Can you work these out from the model? Positions are in its coordinate system, mm. Face numbers are marked on the shaded views. Give positions to 0.01 mm unless a question says otherwise; leave off trailing zeros. Order: outer loops, then holes, each group sorted by start corner. A loop starts at its lowest first (then second) coordinate and runs counter-clockwise, first axis right, second up. Notation, with made-up numbers: (31.25, 31.25) - (46.25, 31.25) arc R29 ccw to (46.25, 70.25) - close; hole circle Ø4 at (79, -18). An arc over 180 degrees is marked (long way). Use one line per item in the form item = value. Start each with the question number.
1) Please list where these lines run through material, in increasing order: probe 1 along Z at (x, y) = (-10, 3.7); probe 2 along X at (y, z) = (1.4, -10).
2) We'd pull the mould along Z, two halves only. Please class the marked faces 1, 2 and 3: released by +Z, released by -Z, zero draft, split by the parting line, or undercut.
3) For pin 1 (3 mm diameter, centred on x = -7.5, z = -1, fed in from -Y), with a flat end and sliding along its axis, tell me the tip position at first contact or that it passes through.
4) Suppose I cut it at A-A, the plane y = 3.55. Write out the boundary of the cut face in (x, z).
Autodesk Fusion 360 part; units mm, degrees
sketch "Skizze1" plane through (0, 0, 0) normal (0, 1, 0) x (1, 0, 0)
  line L0 (10, 10) -> (-10, 10) construction
  line L1 (-10, 10) -> (-10, -10) construction
  line L2 (-10, -10) -> (10, -10) construction
  line L3 (10, -10) -> (10, 10) construction
  line L4 (10, 10) -> (-10, -10) construction
  line L5 (-10, 10) -> (10, -10) construction
  circle A0 centre (-10, 10) radius 0.8
  circle A1 centre (10, 10) radius 0.8
  circle A2 centre (10, -10) radius 0.8
  circle A3 centre (-10, -10) radius 0.8
  line L6 (12, 12) -> (-12, 12)
  line L7 (-12, 12) -> (-12, -12)
  line L8 (-12, -12) -> (12, -12)
  line L9 (12, -12) -> (12, 12)
  line L10 (12, 12) -> (-12, -12) construction
  line L11 (-12, 12) -> (12, -12) construction
  circle A4 centre (0, 0) radius 9
  dimension "d1" = 20
  dimension "d2" = 20
  dimension "d3" = 1.6
  dimension "d4" = 24
  dimension "d16" = 18
extrude "Extrusion1" add sketch "Skizze1" along normal blind 4
sketch "Skizze2" plane through (0, 0, 12) normal (0, 0, 1) x (1, 0, 0)
  line L0 (-12, 0) -> (12, 0)
  line L1 (12, 4) -> (-12, 4)
  line L2 (-12, 4) -> (-12, 0)
  ellipse E0 centre (0, 0) end of major axis (8, 0) minor radius 2.5
  line L3 (-8, 0) -> (8, 0)
  line L4 (0, -2.5) -> (0, 2.5)
  dimension "d8" = 16
  dimension "d9" = 5
extrude "Extrusion2" cut sketch "Skizze2" against normal blind 27 contours L0 E0 L3 L4 | L0 E0 L3 L4 picked at (-4.5024, 0.6044) picked at (4.5261, 0.5973)
sketch "Skizze3" plane through (12, 0, 0) normal (1, 0, 0) x (0, 0, -1)
  line L0 (-12, 0) -> (12, 0)
  line L1 (12, 0) -> (12, 4)
  line L2 (12, 4) -> (-12, 4)
  line L3 (-12, 4) -> (-12, 0)
  ellipse E0 centre (0, 0) end of major axis (8, 0) minor radius 2.5
  line L4 (-8, 0) -> (8, 0)
  line L5 (0, -2.5) -> (0, 2.5)
  dimension "d12" = 5
  dimension "d13" = 16
extrude "Extrusion3" cut sketch "Skizze3" against normal blind 27 contours L0 E0 L4 L5 | L0 E0 L4 L5 picked at (-4.5024, 0.6044) picked at (4.5261, 0.5973)
fillet "Abrundung1" radius 2 4 edges at (12, 2, -12) (-12, 2, 12) (-12, 2, -12) (12, 2, 12)
equation "d1 = d2"
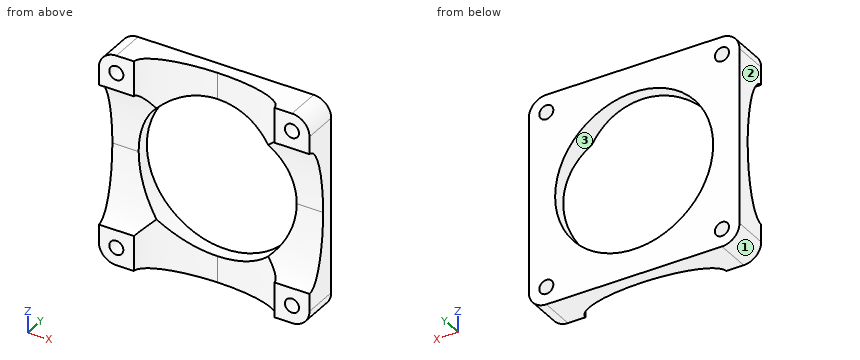
Result sheet:
q1.probe_1 = -12 to -10.8, -9.2 to 9.2, 10.8 to 12
q1.probe_2 = -12 to -10.8, -9.2 to -6.63, 6.63 to 9.2, 10.8 to 12
q2.face_1 = released by -Z
q2.face_2 = zero draft
q2.face_3 = undercut
q3.pin_1 = 2.45
q4.outline = (-12, -10) arc R2 ccw to (-10, -12) - (10, -12) arc R2 ccw to (12, -10) - (12, 10) arc R2 ccw to (10, 12) - (-10, 12) arc R2 ccw to (-12, 10) - close; hole circle Ø1.6 at (-10, -10); hole circle Ø1.6 at (-10, 10); hole circle Ø18 at (0, 0); hole circle Ø1.6 at (10, -10); hole circle Ø1.6 at (10, 10)
